Input: part model. Units: mm. Frame: model coordinates. Face numbers are marked on the shaded views. A direction names the side the tool comes from. Give positions to 0.01 mm unless a question says otherwise; leave off trailing zeros. Write each loop counter-clockwise with the first axis right and the second up, starting at its lowest first coordinate (ties: lowest second). Pieces come first, ordered by that corner, then holes.
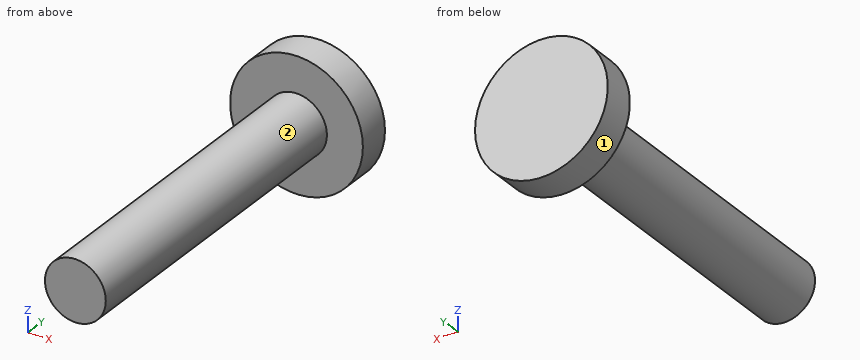
```python
from build123d import *

# Parameters (mm, degrees)
SKETCH1_R           = 10
BOSS_EXTRUDE1_DEPTH = 90
SCALE_1_SCALE       = 0.3
SKETCH_1_R          = 6
EXTRUDE_1_DEPTH     = 3
SKETCH_2_R          = 3
EXTRUDE_3_DEPTH     = 3
SKETCH_3_R          = 3
SKETCH_3_R_2        = 2.75
CUT_EXTRUDE_2_DEPTH = 30


with BuildPart() as part:
    # Sketch1 → Boss-Extrude1 (new body)
    with BuildSketch(Plane(origin=(0, 0, 0), x_dir=(1, 0, 0), z_dir=(0, 1, 0))):
        Circle(SKETCH1_R)
    extrude(amount=BOSS_EXTRUDE1_DEPTH)


with BuildPart() as part_1:
    # 축척1: scaled about (0, 45, 0)
    add(part.part.scale(SCALE_1_SCALE).moved(Location((0, 31.5, 0))))

    # 스케치1 → 보스-돌출1 (add)
    with BuildSketch(Plane(origin=(0, 58.5, 0), x_dir=(1, 0, 0), z_dir=(0, 1, 0))):
        Circle(SKETCH_1_R)
    extrude(amount=EXTRUDE_1_DEPTH)

    # 스케치2 → 보스-돌출3 (add)
    with BuildSketch(Plane.XZ.offset(-31.5)):
        Circle(SKETCH_2_R)
    extrude(amount=EXTRUDE_3_DEPTH)

    # 스케치3 → 컷-돌출2 (cut)
    with BuildSketch(Plane.XZ.offset(-28.5)):
        Circle(SKETCH_3_R)
        Circle(SKETCH_3_R_2, mode=Mode.SUBTRACT)
    extrude(amount=-CUT_EXTRUDE_2_DEPTH, mode=Mode.SUBTRACT)


solid = part_1.part
```
Q1. Section B-B, the plane x = 0. Return the cut outline in (y, z), then the cut area to 3 significant figures.
Q2. Access query for the marked faces 1 and 2. Directions: +Z, -Z, +X, -X, +Y, -Y. A direction counts if a zero-diameter tool reaches every point of the face in a straight line with its end or side. Return the directions, or none.
Q3. Material intervals for line 1 along Y through (x, z) = (-5.5, -1.25); line 2 along Z through (x, y) = (0, 41); line 3 along Z through (x, y) = (-4.75, 59.5), sorted ascending.
Q4. Section D-D, the plane z = -3.25. Return the cut outline in (x, y).
Q5. Section C-C, the plane y = 37. Return the cut outline in (x, z).
Q6. Pin query (flat end, axial travel): pin 1 (1.5 mm diameter, centred on x = -2.5, y = 50, fed in from +Z); pin 2 (4 mm diameter, centred on x = 3, z = 2.5, fed in from -Y); pin 3 (5 mm diameter, centred on y = 49, z = 1.5, fed in from -X); pin 4 (2 mm diameter, centred on x = -1, z = 4.5, fed in from -Y). Return the tip coordinate at first contact, or that it passes through.
Q7. Section A-A, the plane z = 0. Return the cut outline in (x, y).
Solutions:
1. outline: (28.5, -2.75) - (58.5, -2.75) - (58.5, -6) - (61.5, -6) - (61.5, 6) - (58.5, 6) - (58.5, 2.75) - (28.5, 2.75) - close
1. area: 201 mm2
2. face 1: +Y, -Y
2. face 2: -Y
3. line 1: y = 58.5 to 61.5
3. line 2: z = -2.75 to 2.75
3. line 3: z = -3.67 to 3.67
4. outline: (-5.04, 58.5) - (5.04, 58.5) - (5.04, 61.5) - (-5.04, 61.5) - close
5. outline: circle Ø5.5 at (0, 0)
6. pin 1: stops at z = 2.12
6. pin 2: stops at y = 28.5
6. pin 3: stops at x = -2.75
6. pin 4: stops at y = 58.5
7. outline: (-6, 58.5) - (-2.75, 58.5) - (-2.75, 28.5) - (2.75, 28.5) - (2.75, 58.5) - (6, 58.5) - (6, 61.5) - (-6, 61.5) - close
